from build123d import *

# Parameters (mm, degrees)
BOSS_EXTRUDE2_DEPTH     = 10
BOSS_EXTRUDE3_DEPTH     = 2
SKETCH3_R               = 5.825
CUT_EXTRUDE1_DEPTH      = 2
BOSS_EXTRUDE4_START     = 12
SKETCH4_R               = 8.825
SKETCH4_R_2             = 5.825
BOSS_EXTRUDE4_DEPTH     = 12
CUT_EXTRUDE2_DEPTH      = 33.125068093
CUT_EXTRUDE2_DEPTH_BACK = 33.125068093
SKETCH5_R               = 1.5
CHAMFER1_SIZE           = 1


with BuildPart() as part:
    # Sketch1 → Boss-Extrude2 (new body)
    with BuildSketch(Plane(origin=(0, 0, 0), x_dir=(0, 0, -1), z_dir=(1, 0, 0))):
        with BuildLine():
            Line((-11.595322565, 6.716285775), (-12.834408967, 7.955372177))
            ThreePointArc((-12.834408967, 7.955372177), (-15.1, 0), (-12.834408967, -7.955372177))
            Line((-12.834408967, -7.955372177), (-11.595322565, -6.716285775))
            ThreePointArc((-11.595322565, -6.716285775), (-9.475230868, -9.475230868), (-6.716285775, -11.595322565))
            Line((-6.716285775, -11.595322565), (-7.955372177, -12.834408967))
            ThreePointArc((-7.955372177, -12.834408967), (0, -15.1), (7.955372177, -12.834408967))
            Line((7.955372177, -12.834408967), (6.716285775, -11.595322565))
            ThreePointArc((6.716285775, -11.595322565), (9.475230868, -9.475230868), (11.595322565, -6.716285775))
            Line((11.595322565, -6.716285775), (12.834408967, -7.955372177))
            ThreePointArc((12.834408967, -7.955372177), (14.522561334, -4.135844811), (15.1, 0))
            ThreePointArc((15.1, 0), (14.522561334, 4.135844811), (12.834408967, 7.955372177))
            Line((12.834408967, 7.955372177), (11.595322565, 6.716285775))
            ThreePointArc((11.595322565, 6.716285775), (9.475230868, 9.475230868), (6.716285775, 11.595322565))
            Line((6.716285775, 11.595322565), (7.955372177, 12.834408967))
            ThreePointArc((7.955372177, 12.834408967), (0, 15.1), (-7.955372177, 12.834408967))
            Line((-7.955372177, 12.834408967), (-6.716285775, 11.595322565))
            ThreePointArc((-6.716285775, 11.595322565), (-9.475230868, 9.475230868), (-11.595322565, 6.716285775))
        make_face()
        with BuildLine():
            Line((-11.330679795, 5.037429442), (-12.607267332, 6.31401698))
            ThreePointArc((-12.607267332, 6.31401698), (-14.1, 0), (-12.607267332, -6.31401698))
            Line((-12.607267332, -6.31401698), (-11.330679795, -5.037429442))
            ThreePointArc((-11.330679795, -5.037429442), (-8.768124087, -8.768124087), (-5.037429442, -11.330679795))
            Line((-5.037429442, -11.330679795), (-6.31401698, -12.607267332))
            ThreePointArc((-6.31401698, -12.607267332), (0, -14.1), (6.31401698, -12.607267332))
            Line((6.31401698, -12.607267332), (5.037429442, -11.330679795))
            ThreePointArc((5.037429442, -11.330679795), (8.768124087, -8.768124087), (11.330679795, -5.037429442))
            Line((11.330679795, -5.037429442), (12.607267332, -6.31401698))
            ThreePointArc((12.607267332, -6.31401698), (13.721743136, -3.244035343), (14.1, 0))
            ThreePointArc((14.1, 0), (13.721743136, 3.244035343), (12.607267332, 6.31401698))
            Line((12.607267332, 6.31401698), (11.330679795, 5.037429442))
            ThreePointArc((11.330679795, 5.037429442), (8.768124087, 8.768124087), (5.037429442, 11.330679795))
            Line((5.037429442, 11.330679795), (6.31401698, 12.607267332))
            ThreePointArc((6.31401698, 12.607267332), (0, 14.1), (-6.31401698, 12.607267332))
            Line((-6.31401698, 12.607267332), (-5.037429442, 11.330679795))
            ThreePointArc((-5.037429442, 11.330679795), (-8.768124087, 8.768124087), (-11.330679795, 5.037429442))
        make_face(mode=Mode.SUBTRACT)
    extrude(amount=BOSS_EXTRUDE2_DEPTH)

    # Sketch2 → Boss-Extrude3 (add)
    with BuildSketch(Plane(origin=(10, 0, 0), x_dir=(0, 0, -1), z_dir=(1, 0, 0))):
        with BuildLine():
            Line((-12.834408967, -7.955372177), (-11.595322565, -6.716285775))
            ThreePointArc((-11.595322565, -6.716285775), (-9.475230868, -9.475230868), (-6.716285775, -11.595322565))
            Line((-6.716285775, -11.595322565), (-7.955372177, -12.834408967))
            ThreePointArc((-7.955372177, -12.834408967), (0, -15.1), (7.955372177, -12.834408967))
            Line((7.955372177, -12.834408967), (6.716285775, -11.595322565))
            ThreePointArc((6.716285775, -11.595322565), (9.475230868, -9.475230868), (11.595322565, -6.716285775))
            Line((11.595322565, -6.716285775), (12.834408967, -7.955372177))
            ThreePointArc((12.834408967, -7.955372177), (15.1, 0), (12.834408967, 7.955372177))
            Line((12.834408967, 7.955372177), (11.595322565, 6.716285775))
            ThreePointArc((11.595322565, 6.716285775), (9.475230868, 9.475230868), (6.716285775, 11.595322565))
            Line((6.716285775, 11.595322565), (7.955372177, 12.834408967))
            ThreePointArc((7.955372177, 12.834408967), (0, 15.1), (-7.955372177, 12.834408967))
            Line((-7.955372177, 12.834408967), (-6.716285775, 11.595322565))
            ThreePointArc((-6.716285775, 11.595322565), (-9.475230868, 9.475230868), (-11.595322565, 6.716285775))
            Line((-11.595322565, 6.716285775), (-12.834408967, 7.955372177))
            ThreePointArc((-12.834408967, 7.955372177), (-15.1, 0), (-12.834408967, -7.955372177))
        make_face()
    extrude(amount=BOSS_EXTRUDE3_DEPTH)

    # Sketch3 → Cut-Extrude1 (cut)
    with BuildSketch(Plane(origin=(12, 0, 0), x_dir=(0, 0, -1), z_dir=(1, 0, 0))):
        Circle(SKETCH3_R)
    extrude(amount=-CUT_EXTRUDE1_DEPTH, mode=Mode.SUBTRACT)

    # Sketch4 → Boss-Extrude4 (add)
    with BuildSketch(Plane(origin=(12, 0, 0), x_dir=(0, 0, -1), z_dir=(1, 0, 0)).offset(BOSS_EXTRUDE4_START)):
        Circle(SKETCH4_R)
        Circle(SKETCH4_R_2, mode=Mode.SUBTRACT)
    extrude(amount=-BOSS_EXTRUDE4_DEPTH)

    # Sketch5 → Cut-Extrude2 (cut, two sides: drawn at the far end of the back side and taken through both)
    with BuildSketch(Plane(origin=(0, 0, 0), x_dir=(1, 0, 0), z_dir=(0, 1, 0)).offset(-CUT_EXTRUDE2_DEPTH_BACK)):
        with Locations(Location((16, 0, 0), (0, 0, 270))):
            Circle(SKETCH5_R)
    extrude(amount=CUT_EXTRUDE2_DEPTH + CUT_EXTRUDE2_DEPTH_BACK, mode=Mode.SUBTRACT)

    # Chamfer1
    chamfer1_edges = [part.edges().sort_by_distance(p)[0] for p in [
        (10, 0, 5.825),
    ]]
    chamfer(chamfer1_edges, length=CHAMFER1_SIZE)


solid = part.part
Work out the finished part from the listing and answer in its coordinate system (mm). A direction names the side the tool comes from. Give positions to 0.01 mm unless a question says otherwise; leave off trailing zeros. Loops run counter-clockwise (first coordinate to the right, second up) from the corner with the lowest first, then second, coordinate; pieces in that order, holes last. Notation, with made-up numbers: M 6.5,54.25 L 13.5,54.25 A34 ccw 13.5,86.25 Z; hole C 65.5,81 d11. An arc over 180 degrees is marked long. Use CSV: the item, a comma, the result in double quotes.
1) Find section C-C on x = 16. Write down the section's boundary in (y, z) (3 decimals).
Answer:
outline,"M -8.697,-1.5 A8.825 ccw 8.697,-1.5 L 5.629,-1.5 A5.825 cw -5.629,-1.5 Z; M -8.697,1.5 L -5.629,1.5 A5.825 cw 5.629,1.5 L 8.697,1.5 A8.825 ccw Z"
2) Find section A-A on z = 0. Write down the section's boundary in (x, y) (3 decimals), plus the area to 3 significant figures.
Answer:
outline,"M 0,-15.1 L 12,-15.1 L 12,-8.825 L 14.5,-8.825 L 14.5,-5.825 L 11,-5.825 L 10,-6.825 L 10,-14.1 L 0,-14.1 Z; M 0,14.1 L 10,14.1 L 10,6.825 L 11,5.825 L 14.5,5.825 L 14.5,8.825 L 12,8.825 L 12,15.1 L 0,15.1 Z; M 17.5,-8.825 L 24,-8.825 L 24,-5.825 L 17.5,-5.825 Z; M 17.5,5.825 L 24,5.825 L 24,8.825 L 17.5,8.825 Z"
area,"110 mm^2"
3) Find section D-D on y = -10. Write down the section's boundary in (x, z).
Answer:
outline,"M 0,-8.92 L 12,-8.92 L 12,8.92 L 0,8.92 L 0,7.33 L 10,7.33 L 10,-7.33 L 0,-7.33 Z"
4) Determine the mould class of faces 4 (the cylindrical face through (18.084, -8.615, 1.913)), 5 (the cylindrical face through (17.265, -7.248, 0.806)), 6 (the flat face through (4.93, -5.685, 11.978)) for opening direction Y: released by +Y, released by -Y, zero draft, split by the parting line, or undercut.
Answer:
face 4,"split by the parting line"
face 5,"zero draft"
face 6,"undercut"
5) Which of the six approach directions +Z, -Z, +X, -X, +Y, -Y give full straight-line access (tool end or side, diameter ignored) to faces 1 (the flat face through (5.92, -12.21, 7.33)), 2 (the flat face through (4.93, 11.978, 5.685)), 3 (the flat face through (5.92, -12.22, -7.34))?
Answer:
face 1,"+Z, +X, -X"
face 2,"-X"
face 3,"-Z, +X, -X"
6) Given P1, Ø5, axis at x = 10, y = 12, coming from the -Z side; P2, Ø10, axis at x = 21, y = 11, coming from the -Z side; P3, Ø5, axis at x = 16, z = 0, coming from the -Y side (3 decimals); P4, Ø12, axis at y = -12, z = 5, coming from the +X side, each flat-ended and moving along its own axis, determine where each tip first touches the part or whether it passes through.
Answer:
P1,"z = -9.45"
P2,"z = -6.47"
P3,"y = -8.825"
P4,"x = 24"
7) Consider L1, parallel to Y at x = 20.75, z = 0 (3 decimals); L2, parallel to Y at x = 6.25, z = -0.5; L3, parallel to Z at x = 1.5, y = -7.5. Determine where each line is inside the solid, lowest interval first.
Answer:
L1,"-8.825 to -5.825, 5.825 to 8.825"
L2,"-15.09 to -14.09, 14.09 to 15.09"
L3,"-13.11 to -12.38, -11.1 to -9.87, 9.87 to 11.1, 12.38 to 13.11"
